Source: CAD feature listing. Evaluate the final solid. Frame: model axes, mm. A direction names the side the tool comes from. Give positions to 0.01 mm unless a question says otherwise; leave off trailing zeros. Loops run counter-clockwise (first coordinate to the right, second up) from the corner with the lowest first, then second, coordinate; pieces in that order, holes last. Notation, with made-up numbers: (45.5, 41) -> (76.5, 41) arc R15 cw to (76.5, 54) -> close; hole circle Ø11 at (36.5, 63). An arc over 180 degrees is marked (long way). Put each result on its own line as item: value.
```python
from build123d import *

# Parameters (mm, degrees)
SKETCH1_R           = 3.175
BOSS_EXTRUDE1_DEPTH = 60
SKETCH2_R           = 4
CUT_EXTRUDE1_DEPTH  = 61
BOSS_EXTRUDE2_DEPTH = 60
SKETCH5_W           = 5.08
SKETCH5_H           = 8.6
BOSS_EXTRUDE3_DEPTH = 21.1
CUT_EXTRUDE2_REACH  = 54.578
SKETCH6_R           = 1.25
FILLET1_R           = 2.54
FILLET3_R           = 5.08
FILLET4_R           = 5.08


with BuildPart() as part:
    # Sketch1 → Boss-Extrude1 (new body)
    with BuildSketch(Plane.XY):
        with BuildLine():
            Line((0, 0), (41.801331845, 0))
            Line((41.801331845, 0), (43.146541753, 12.096417759))
            ThreePointArc((43.146541753, 12.096417759), (38.021254436, 18.152629022), (32.258, 12.7))
            Line((32.258, 12.7), (32.258, 6.35))
            Line((32.258, 6.35), (0, 6.35))
            Line((0, 6.35), (0, 0))
        make_face()
        with Locations((37.719, 12.7)):
            Circle(SKETCH1_R, mode=Mode.SUBTRACT)
    boss_extrude1 = extrude(amount=BOSS_EXTRUDE1_DEPTH)

    # Sketch2 → Cut-Extrude1 (cut, through all)
    with BuildSketch(Plane(origin=(0, 0, 0), x_dir=(-1, 0, 0), z_dir=(0, 0, -1))):
        with Locations((0, -2.54)):
            Circle(SKETCH2_R)
    cut_extrude1 = extrude(amount=-CUT_EXTRUDE1_DEPTH, mode=Mode.SUBTRACT)

    # Sketch3 → Boss-Extrude2 (add)
    with BuildSketch(Plane(origin=(0, 0, 0), x_dir=(-1, 0, 0), z_dir=(0, 0, -1))):
        with BuildLine():
            Line((-7.385424835, 0), (-3.090048543, 0))
            ThreePointArc((-3.090048543, 0), (-3.616628264, -4.248800749), (0, -6.54))
            Line((0, -6.54), (0, -10.35))
            ThreePointArc((0, -10.35), (-6.357416928, -7.076446847), (-7.385424835, 0))
        make_face()
    boss_extrude2 = extrude(amount=-BOSS_EXTRUDE2_DEPTH)

    # Mirror1: Boss-Extrude1, Cut-Extrude1, Boss-Extrude2 across plane
    add(boss_extrude1.mirror(Plane(origin=(0, 0, 0), x_dir=(0, 0, 1), z_dir=(1, 0, 0))))
    add(cut_extrude1.mirror(Plane(origin=(0, 0, 0), x_dir=(0, 0, 1), z_dir=(1, 0, 0))), mode=Mode.SUBTRACT)
    add(boss_extrude2.mirror(Plane(origin=(0, 0, 0), x_dir=(0, 0, 1), z_dir=(1, 0, 0))))

    # Sketch5 → Boss-Extrude3 (add)
    with BuildSketch(Plane(origin=(0, 6.35, 0), x_dir=(1, 0, 0), z_dir=(0, 1, 0))):
        with Locations((6.858, -4.3)):
            Rectangle(SKETCH5_W, SKETCH5_H)
        with Locations((6.858, -55.7)):
            Rectangle(SKETCH5_W, SKETCH5_H)
    extrude(amount=BOSS_EXTRUDE3_DEPTH)

    # Sketch6 → Cut-Extrude2 (cut, up to next)
    with BuildSketch(Plane(origin=(9.398, 0, 0), x_dir=(0, 0, -1), z_dir=(1, 0, 0)), mode=Mode.PRIVATE) as cut_extrude2_sk1:
        with Locations((-54.75, 22.4)):
            Circle(SKETCH6_R)
    cut_extrude2_tool1 = extrude(cut_extrude2_sk1.sketch, amount=-CUT_EXTRUDE2_REACH, mode=Mode.PRIVATE) & part.part
    add(cut_extrude2_tool1.solids().sort_by_distance((9.398, 22.4, 54.75))[0], mode=Mode.SUBTRACT)
    # Sketch6 → Cut-Extrude2 (cut, up to next)
    with BuildSketch(Plane(origin=(9.398, 0, 0), x_dir=(0, 0, -1), z_dir=(1, 0, 0)), mode=Mode.PRIVATE) as cut_extrude2_sk2:
        with Locations((-5.25, 22.4)):
            Circle(SKETCH6_R)
    cut_extrude2_tool2 = extrude(cut_extrude2_sk2.sketch, amount=-CUT_EXTRUDE2_REACH, mode=Mode.PRIVATE) & part.part
    add(cut_extrude2_tool2.solids().sort_by_distance((9.398, 22.4, 5.25))[0], mode=Mode.SUBTRACT)
    # Sketch6 → Cut-Extrude2 (cut, up to next)
    with BuildSketch(Plane(origin=(9.398, 0, 0), x_dir=(0, 0, -1), z_dir=(1, 0, 0)), mode=Mode.PRIVATE) as cut_extrude2_sk3:
        with Locations((-5.25, 12.4)):
            Circle(SKETCH6_R)
    cut_extrude2_tool3 = extrude(cut_extrude2_sk3.sketch, amount=-CUT_EXTRUDE2_REACH, mode=Mode.PRIVATE) & part.part
    add(cut_extrude2_tool3.solids().sort_by_distance((9.398, 12.4, 5.25))[0], mode=Mode.SUBTRACT)
    # Sketch6 → Cut-Extrude2 (cut, up to next)
    with BuildSketch(Plane(origin=(9.398, 0, 0), x_dir=(0, 0, -1), z_dir=(1, 0, 0)), mode=Mode.PRIVATE) as cut_extrude2_sk4:
        with Locations((-54.75, 12.4)):
            Circle(SKETCH6_R)
    cut_extrude2_tool4 = extrude(cut_extrude2_sk4.sketch, amount=-CUT_EXTRUDE2_REACH, mode=Mode.PRIVATE) & part.part
    add(cut_extrude2_tool4.solids().sort_by_distance((9.398, 12.4, 54.75))[0], mode=Mode.SUBTRACT)

    # Fillet1
    fillet1_edges = [part.edges().sort_by_distance(p)[0] for p in [
        (9.398, 6.35, 55.7),
        (9.398, 6.35, 4.3),
    ]]
    fillet(fillet1_edges, radius=FILLET1_R)

    # Fillet3
    fillet3_edges = [part.edges().sort_by_distance(p)[0] for p in [
        (7.385424835, 0, 30),
        (-7.385424835, 0, 30),
    ]]
    fillet(fillet3_edges, radius=FILLET3_R)

    # Fillet4
    fillet4_edges = [part.edges().sort_by_distance(p)[0] for p in [
        (41.801331845, 0, 30),
        (-41.801331845, 0, 30),
    ]]
    fillet(fillet4_edges, radius=FILLET4_R)


solid = part.part
```
(1) Section A-A on z = 5.25. Give the number of separate pieces and of enclosed holes in the cut face, then the cut area to 3 significant figures.
Calculated:
separate pieces: 3
enclosed holes: 3
area: 869 mm²
(2) Section D-D on x = 35.5. Return loops of the section in (y, z), then the cut area to 3 significant figures.
Calculated:
outline: (0, 0) -> (10.43, 0) -> (10.43, 60) -> (0, 60) -> close; (14.97, 0) -> (17.69, 0) -> (17.69, 60) -> (14.97, 60) -> close
area: 789 mm²
(3) Line query: probe 1 along X at (y, z) = (12.5, 29.5); probe 2 along X at (y, z) = (12, 37); probe 3 along X at (y, z) = (15, 4.5). Output: solid intervals per line, ascending. Write a range as from..to.
Calculated:
probe 1: x = -43.18..-40.89, -34.55..-32.26, 32.26..34.55, 40.89..43.18
probe 2: x = -43.14..-40.82, -34.62..-32.26, 32.26..34.62, 40.82..43.14
probe 3: x = -42.67..-39.91, -35.53..-32.77, 4.32..9.4, 32.77..35.53, 39.91..42.67
(4) First-contact query: P1, Ø12, axis at y = 6.5, z = 36, coming from the -X side; P2, Ø3, axis at y = 22.4, z = 54.75, coming from the -X side; P3, Ø2.5, axis at y = 15.5, z = 56.5, coming from the -X side; P4, Ø4, axis at y = 20.5, z = 28.5, coming from the -X side. Flat tips, straight axial feed; report the tip coordinate or a pass-through.
Calculated:
P1: stops at x = -43.18
P2: stops at x = 4.32
P3: stops at x = -42.96
P4: passes through
(5) Draft query along Z for faces 6 (the cylindrical face through (40.65, 11.48, 29.58)), 7 (the cylindrical face through (6.89, 12.78, 53.56)). Return one class per face: released by +Z, released by -Z, zero draft, split by the parting line, or undercut.
Calculated:
face 6: zero draft
face 7: undercut
(6) Section C-C on z = 48. Return loops of the section in (x, y) (3 decimals).
Calculated:
outline: (-43.147, 12.096) -> (-42.304, 4.519) arc R5.08 ccw to (-37.255, 0) -> (-12.637, 0) arc R5.08 cw to (-7.657, -4.079) arc R7.81 ccw to (7.657, -4.079) arc R5.08 cw to (12.637, 0) -> (37.255, 0) arc R5.08 ccw to (42.304, 4.519) -> (43.147, 12.096) arc R5.461 ccw (long way) to (32.258, 12.7) -> (32.258, 6.35) -> (-32.258, 6.35) -> (-32.258, 12.7) arc R5.461 ccw (long way) to start; hole circle Ø6.35 at (-37.719, 12.7); hole circle Ø8 at (0, -2.54); hole circle Ø6.35 at (37.719, 12.7)
(7) Reachability of faces 1 (the flat face through (7, 17, 51.4)), 2 (the flat face through (42.72, 8.25, 29.58)), 3 (the flat face through (-25, 0, 30)), 4 (the flat face through (4.318, 17, 4)), 5 (the cylindrical face through (6.894, 23.245, 6.171)) from +Z, -Z, +X, -X, +Y, -Y: full face, straight path, thin tool, end or side. Return the list, or none.
Calculated:
face 1: +Y
face 2: +Z, -Z, +X, -Y
face 3: +Z, -Z, -X, -Y
face 4: +Z, -Z, +Y
face 5: +X, -X
(8) Section B-B on y = 22.4. Return loops of the section in (x, z), then the cut area to 3 significant figures.
Calculated:
outline: (4.32, 0) -> (9.4, 0) -> (9.4, 4) -> (4.32, 4) -> close; (4.32, 6.5) -> (9.4, 6.5) -> (9.4, 8.6) -> (4.32, 8.6) -> close; (4.32, 51.4) -> (9.4, 51.4) -> (9.4, 53.5) -> (4.32, 53.5) -> close; (4.32, 56) -> (9.4, 56) -> (9.4, 60) -> (4.32, 60) -> close
area: 62.0 mm²
